from build123d import *

# Parameters (mm, degrees)
F0_R     = 30
F1_DEPTH = 48
F3_R     = 10
F4_DEPTH = 10
F6_R     = 10
F7_DEPTH = 10


with BuildPart() as f1:
    # F0 (on Right) → F1 (new body)
    with BuildSketch(Plane.YZ):
        Circle(F0_R)
    extrude(amount=F1_DEPTH)

    # F3 (on offset) → F4 (cut)
    with BuildSketch(Plane.XZ.offset(30)):
        with Locations((13, 0)):
            Circle(F3_R)
    extrude(amount=-F4_DEPTH, mode=Mode.SUBTRACT)

    # F6 (on offset) → F7 (cut)
    with BuildSketch(Plane.XZ.offset(-30)):
        with Locations((13, 0)):
            Circle(F6_R)
    extrude(amount=F7_DEPTH, mode=Mode.SUBTRACT)


solid = f1.part
Source: CAD feature listing. Evaluate the final solid. Frame: model axes, mm. A direction names the side the tool comes from. Give positions to 0.01 mm unless a question says otherwise; leave off trailing zeros. Write each loop counter-clockwise with the first axis right and the second up, starting at its lowest first coordinate (ties: lowest second). Pieces come first, ordered by that corner, then holes. Notation, with made-up numbers: M 13,40 L 64,40 A22 cw 64,53 Z; hole C 33,35.25 d9. An arc over 180 degrees is marked long. Return JSON: item names as keys, results as strings. Group by question number.
1) Cut plane D-D, the plane y = 25.5. Output: boundary loops of the cut face in (x, z), then the cut area to 3 significant figures.
2) Ray query, L1, parallel to X at y = -28, z = 0; L2, parallel to Z at x = 13, y = 22.5; L3, parallel to Z at x = 13, y = -21.75. Return the intervals inside material, ascending.
3) Cut plane C-C, the plane y = -18. Output: boundary loops of the cut face in (x, z), then the cut area to 3 significant figures.
4) First-contact query: pin 1 Ø12 at (x, z) = (13, 0) entering from -Y; pin 2 Ø1 at (x, z) = (23.5, 9) entering from -Y; pin 3 Ø2 at (x, y) = (35, -9.5) entering from -Z. Flat tips, straight axial feed; report the tip coordinate or a pass-through.
5) Draft query along X for faces 1 (the face through (0, 0, 0)), 2 (the face through (48, 0, 0)), 3 (the face through (13, 20, 0)). Return one class per face: released by +X, released by -X, zero draft, split by the parting line, or undercut.
6) Set-up query: faces 4 (the face through (22.54, -25.07, 3)), 5 (the face through (23.664, 27.712, -11.49)), 6 (the face through (22.54, 25.07, 3)). Return all of +Z, -Z, +X, -X, +Y, -Y with unobstructed straight access to the full face (end or side cutting, diameter ignored); none if empty.
7) Cut plane B-B, the plane x = 13. Output: boundary loops of the cut face in (y, z).
8) Cut plane A-A, the plane z = 0. Output: boundary loops of the cut face in (x, y).
Data:
{
 "1": {"outline": "M 0,-15.8 L 48,-15.8 L 48,15.8 L 0,15.8 Z; hole C 13,0 d20", "area": "1,200 mm²"},
 "2": {"L1": "x = 0 to 3, 23 to 48", "L2": "z = -19.84 to -10, 10 to 19.84", "L3": "z = -20.66 to -10, 10 to 20.66"},
 "3": {"outline": "M 0,-24 L 48,-24 L 48,24 L 0,24 Z", "area": "2,300 mm²"},
 "4": {"pin 1": "stops at y = -20", "pin 2": "stops at y = -28.77", "pin 3": "stops at z = -28.77"},
 "5": {"face 1": "released by -X", "face 2": "released by +X", "face 3": "undercut"},
 "6": {"face 4": "-Y", "face 5": "+X, -X", "face 6": "+Y"},
 "7": {"outline": "M -28.28,-10 A30 ccw 28.28,-10 L 20,-10 L 20,10 L 28.28,10 A30 ccw -28.28,10 L -20,10 L -20,-10 Z"},
 "8": {"outline": "M 0,-30 L 3,-30 L 3,-20 L 23,-20 L 23,-30 L 48,-30 L 48,30 L 23,30 L 23,20 L 3,20 L 3,30 L 0,30 Z"}
}
